Input: dimensioned drawing with shaded views. Units: mm. Origin: part minimum x, y, z. Coordinates: 2 decimals unless noted, no trailing zeros. Order: outer loops, then holes, each group sorted by start corner. A loop starts at its lowest first (then second) coordinate and runs counter-clockwise, first axis right, second up. Notation, with made-up numbers: (-23, 8) -> (-15, 8) arc R33 ccw to (-15, 41) -> close; hole circle Ø1 at (55, 0.25). An arc over 180 degrees is marked (long way). Answer as CSV lines item,"result".
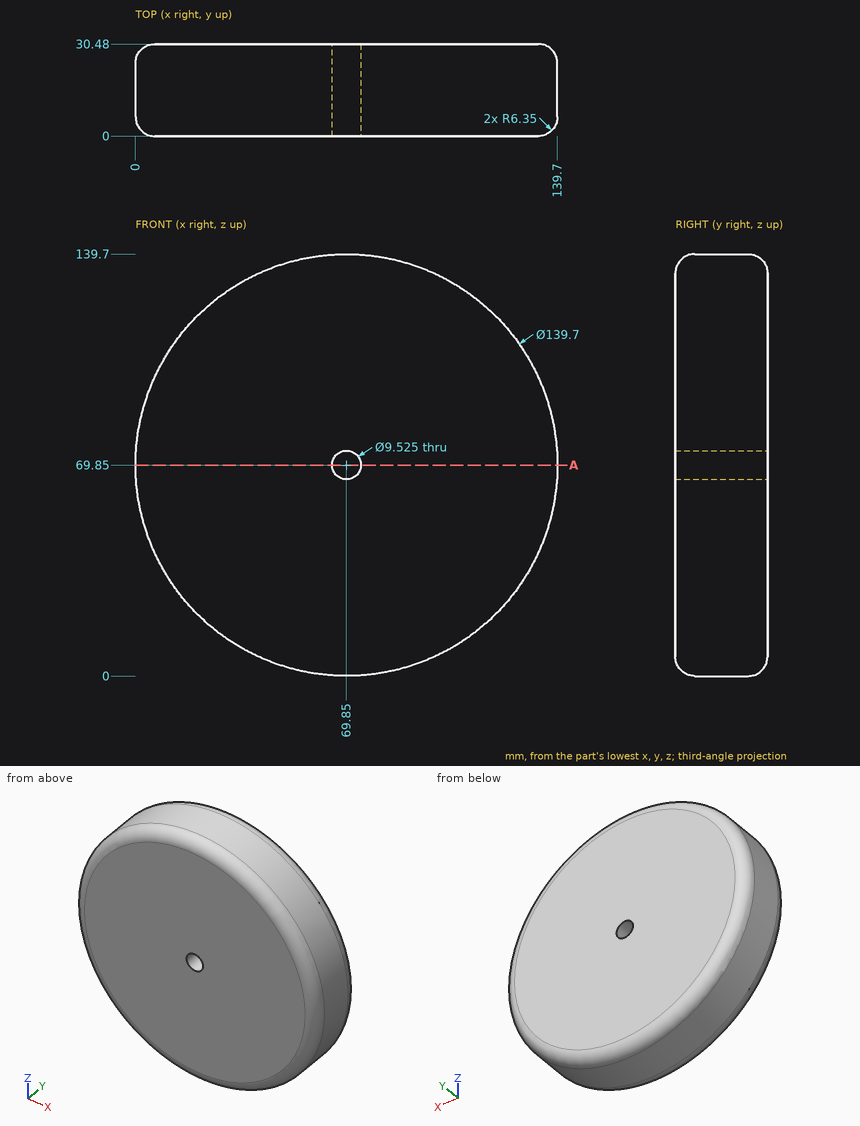
1. Contact query for flat-ended pins moving along their axis: pin 1 (4 mm diameter, centred on x = 62, y = 20.5, fed in from -Z); pin 2 (1 mm diameter, centred on x = 92, z = 47, fed in from -Y); pin 3 (7.5 mm diameter, centred on x = 69.85, z = 69.85, fed in from -Y); pin 4 (12 mm diameter, centred on x = 113.5, y = 20, fed in from +Z). Output: stop coordinate, or through.
Findings:
pin 1,"stops at z = 0.25"
pin 2,"stops at y = 0"
pin 3,"passes through"
pin 4,"stops at z = 128.68"
2. Cut plane A-A (z = 69.85). Return the cut outline in (x, y), plus the area to 3 significant figures.
Findings:
outline,"(0, 6.35) arc R6.35 ccw to (6.35, 0) -> (65.09, 0) -> (65.09, 30.48) -> (6.35, 30.48) arc R6.35 ccw to (0, 24.13) -> close; (74.61, 0) -> (133.35, 0) arc R6.35 ccw to (139.7, 6.35) -> (139.7, 24.13) arc R6.35 ccw to (133.35, 30.48) -> (74.61, 30.48) -> close"
area,"3,930 mm2"
3. Ray query, line 1 along X through (y, z) = (12, 69.85); line 2 along X through (y, z) = (17, 69). Return the intervals inside material, ascending.
Findings:
line 1,"x = 0 to 65.09, 74.61 to 139.7"
line 2,"x = 0.01 to 65.16, 74.54 to 139.69"
